```python
from build123d import *

# Parameters (mm, degrees)
SKETCH2_R          = 21
CUT_EXTRUDE1_DEPTH = 57
SKETCH3_W          = 12
SKETCH3_H          = 8.3
CUT_EXTRUDE2_DEPTH = 57


with BuildPart() as part:
    # Sketch1 → Revolve1 (revolve)
    with BuildSketch(Plane.XY, mode=Mode.PRIVATE) as revolve1_sk:
        Polygon((0, 0), (-13.15, 0), (-13.15, 35), (-23, 44.5), (-23, 122), (-27.5, 122), (-27.5, 185), (-11, 185), (-11, 145), (0, 145), align=None)
    revolve(revolve1_sk.sketch.rotate(Axis((0, 0, 0), (0, 1, 0)), 270), axis=Axis((0, 0, 0), (0, 1, 0)))

    # Sketch2 → Cut-Extrude1 (cut)
    with BuildSketch(Plane(origin=(0, 185, 0), x_dir=(1, 0, 0), z_dir=(0, 1, 0))):
        with Locations(Location((0, 0, 0), (0, 0, 270))):
            Circle(SKETCH2_R)
    extrude(amount=-CUT_EXTRUDE1_DEPTH, mode=Mode.SUBTRACT)

    # Sketch3 → Cut-Extrude2 (cut)
    with BuildSketch(Plane(origin=(0, 185, 0), x_dir=(1, 0, 0), z_dir=(0, 1, 0))):
        with Locations((0, 20.15)):
            Rectangle(SKETCH3_W, SKETCH3_H)
    extrude(amount=-CUT_EXTRUDE2_DEPTH, mode=Mode.SUBTRACT)


solid = part.part
```
The listing builds one solid part. Answer for the finished solid, in the listing's coordinates (mm). A direction names the side the tool comes from. Coordinates: 2 decimals unless noted, no trailing zeros. Loops run counter-clockwise (first coordinate to the right, second up) from the corner with the lowest first, then second, coordinate; pieces in that order, holes last. Notation, with made-up numbers: M -28.75,81 L -22.75,81 A30 cw -22.75,111 Z; hole C 54.5,30 d11. An arc over 180 degrees is marked long. Answer as a JSON object with one key per item and string values. Group by question number.
Item 1: Consider L1, parallel to X at y = 172.5, z = 0; L2, parallel to X at y = 147, z = 5.5; L3, parallel to Y at x = -17, z = 18. Determine where each line is inside the solid, lowest interval first.
Item 2: Determine the mould class of faces 1 (the face through (0, 157, -24.3)), 2 (the face through (-19.394, 83.792, -12.365)), 3 (the face through (20.24, 185, 6.24)) for opening direction Z: +Z half, -Z half, draft (parallel to the pull), parting line (faces both ways), or undercut.
Item 3: Section B-B (z = 0) is taken. Write down the section's boundary in (x, y), and give its area (3 significant figures).
Item 4: Section D-D (y = 26) is taken. Write down the section's boundary in (x, z).
Item 5: Section C-C (y = 77) is taken. Write down the section's boundary in (x, z).
Item 6: Which of the six approach directions +Z, -Z, +X, -X, +Y, -Y give full straight-line access (tool end or side, diameter ignored) to faces 4 (the face through (0, 128, -2)), 5 (the face through (5.037, 17.745, -12.147)), 6 (the face through (0, 0, 0))?
Item 7: Each of these flat-tipped pins is pushed along its axis until it touches: P1, Ø6, axis at x = 8, z = -5, coming from the +Y side; P2, Ø6, axis at y = 43, z = -4.5, coming from the +X side; P3, Ø1.5, axis at x = 19.5, z = 18.5, coming from the -Y side. Where does it stop, or does it pass through?
Item 8: Section A-A (x = 0) is taken. Write down the section's boundary in (y, z), and give its area (3 significant figures).
Solved:
{
 "1": {"L1": "x = -27.5 to -21, 21 to 27.5", "L2": "x = -26.94 to -20.27, 20.27 to 26.94", "L3": "y = 122 to 185"},
 "2": {"face 1": "undercut", "face 2": "parting line", "face 3": "draft"},
 "3": {"outline": "M -27.5,122 L -23,122 L -23,44.5 L -13.15,35 L -13.15,0 L 13.15,0 L 13.15,35 L 23,44.5 L 23,122 L 27.5,122 L 27.5,185 L 21,185 L 21,128 L -21,128 L -21,185 L -27.5,185 Z", "area": "5,900 mm2"},
 "4": {"outline": "C 0,0 d26.3"},
 "5": {"outline": "C 0,0 d46"},
 "6": {"face 4": "+Y", "face 5": "-Y", "face 6": "+Z, -Z, +X, -X, -Y"},
 "7": {"P1": "stops at y = 128", "P2": "stops at x = 22.92", "P3": "stops at y = 122"},
 "8": {"outline": "M 0,-13.15 L 35,-13.15 L 44.5,-23 L 122,-23 L 122,-27.5 L 185,-27.5 L 185,-24.3 L 128,-24.3 L 128,21 L 185,21 L 185,27.5 L 122,27.5 L 122,23 L 44.5,23 L 35,13.15 L 0,13.15 Z", "area": "5,710 mm2"}
}
